Source: CAD feature listing. Evaluate the final solid. Frame: model axes, mm. A direction names the side the tool comes from. Give positions to 0.01 mm unless a question says otherwise; leave off trailing zeros. Write each loop counter-clockwise with the first axis right and the second up, starting at its lowest first coordinate (ties: lowest second). Pieces come first, ordered by that corner, then holes. Notation, with made-up numbers: (-26.5, -24.75) -> (-9.5, -24.75) arc R18 cw to (-9.5, -20.75) -> close; hole circle Ø3 at (14, 66.5). An arc over 180 degrees is marked (long way). Write item = value, one per line.
Autodesk Inventor part; units mm, degrees
ref_plane "YZ Plane" through (0, 0, 0) normal (1, 0, 0) x (0, 1, 0)
ref_plane "XZ Plane" through (0, 0, 0) normal (0, 1, 0) x (-1, 0, 0)
ref_plane "XY Plane" through (0, 0, 0) normal (0, 0, 1) x (1, 0, 0)
sketch "Sketch1" plane through (0, 0, 0) normal (0, 0, 1) x (1, 0, 0)
  line L0 (0, 0) -> (-25.4, 0)
  line L1 (-25.4, 0) -> (-25.4, 25.4)
  line L2 (0, 3.175) -> (-22.225, 3.175)
  line L3 (-22.225, 3.175) -> (-22.225, 25.4)
  line L4 (0, 3.175) -> (0, 0)
  line L5 (-25.4, 25.4) -> (-22.225, 25.4)
  dimension "d0" = 25.4
  dimension "d1" = 25.4
  dimension "d2" = 3.175
extrude "Extrusion1" add sketch "Sketch1" along normal blind 698.5
sketch "Sketch2" plane through (-22.225, 3.175, 0) normal (1, 0, 0) x (0, 0, -1)
  line L0 (0, 22.225) -> (0, 0)
  line L1 (0, 11.1125) -> (0, 6.0325)
  line L2 (0, 6.0325) -> (-85.725, 6.0325)
  line L3 (0, 22.225) -> (-698.5, 22.225)
  line L4 (-349.25, 22.225) -> (-349.25, 11.1125)
  line L5 (-698.5, 22.225) -> (-698.5, 0)
  line L6 (-698.5, 11.1125) -> (-698.5, 6.0325)
  line L7 (-698.5, 6.0325) -> (-612.775, 6.0325)
  line L8 (-698.5, 22.225) -> (0, 22.225)
  point P0 (0, -3.175)
  point P1 (-698.5, -3.175)
  dimension "d5" = 5.08
  dimension "d6" = 85.725
hole "Hole1" at (-22.225, 9.2075, 612.775) at (-22.225, 9.2075, 85.725) direction (-1, 0, 0) diameter 6.35 end through all
properties part number "27.5 L"
(1) First-contact query: pin 1 (3 mm diameter, centred on x = -4, z = 580.5, fed in from +Y) (3 decimals); pin 2 (5 mm diameter, centred on y = 18, z = 170.5, fed in from +X) (3 decimals). Flat tips, straight axial feed; report the tip coordinate or a pass-through.
Values follow:
pin_1 = 3.175
pin_2 = -22.225
(2) Section query A-A (x = -7). Return loops of the section in (y, z) (3 decimals).
Values follow:
outline = (0, 0) -> (3.175, 0) -> (3.175, 698.5) -> (0, 698.5) -> close
(3) Section query B-B (z = 141). Return loops of the section in (x, y) (3 decimals), plus the area to 3 significant figures.
Values follow:
outline = (-25.4, 0) -> (0, 0) -> (0, 3.175) -> (-22.225, 3.175) -> (-22.225, 25.4) -> (-25.4, 25.4) -> close
area = 151 mm2
(4) Material intervals for line 1 (Y direction, x = -18.25, z = 130.5) (3 decimals); line 2 (X direction, y = 11.5, z = 380.5) (3 decimals), sorted ascending.
Values follow:
line_1 = 0 to 3.175
line_2 = -25.4 to -22.225
(5) Section query C-C (y = 20.25). Return loops of the section in (x, z) (3 decimals), plus the area to 3 significant figures.
Values follow:
outline = (-25.4, 0) -> (-22.225, 0) -> (-22.225, 698.5) -> (-25.4, 698.5) -> close
area = 2,220 mm2
(6) Access query for faces 1 (the face through (-22.225, 14, 344)), 2 (the face through (-25.4, 13, 344)). Directions: +Z, -Z, +X, -X, +Y, -Y. A direction counts if a zero-diameter tool reaches every point of the face in a straight line with its end or side. Return the directions, or none.
Values follow:
face_1 = +Z, -Z, +X, +Y
face_2 = +Z, -Z, -X, +Y, -Y
